Could you check a few things on this model? Use its own coordinates, in mm. Give positions to 0.01 mm unless a question says otherwise; leave off trailing zeros. Loops run counter-clockwise (first coordinate to the right, second up) from the corner with the lowest first, then second, coordinate; pieces in that order, holes last. Notation, with made-up numbers: (76.5, 29.25) - (116.5, 29.25) arc R17 ccw to (116.5, 42.25) - close; hole circle Ø5 at (14, -2). An arc over 180 degrees is marked (long way). Write each question's results on one line, items separated by ' | '. Start each with the question number.
1) I want a section at A-A, the plane y = 92.5. Write out the boundary of the cut face in (x, z).
2) I'm going to push a flat-ended pin straight in: pin 1 (3 mm diameter, centred on y = 106.77, z = 239.43, fed in from +X). Where does the tip first touch, or does it pass through?
3) If we mould it in two halves opening along X, with no side actions, what happens to faces 1 (the face through (2, 75, 404.535)), 2 (the face through (4.762, 46, 295)), 3 (the face through (0, 46, 295))? For each: +X half, -X half, draft (parallel to the pull), parting line (faces both ways), or undercut.
4) I want a section at C-C, the plane x = 1.25. Count the separate pieces of the cut face and the enclosed holes in it, and give its area (3 significant figures).
5) I want a section at D-D, the plane y = 82.5. Write out the boundary of the cut face in (x, z), and give its area (3 significant figures).
6) If I drill on probe 1 along Z at (x, y) = (3.6, 42); probe 2 along Z at (x, y) = (2.7, 79); probe 3 along Z at (x, y) = (3.35, 88), over which ranges is the centre line in solid material (lowest first)? Write a range as [from, to].
7) I want a section at B-B, the plane z = 308. Write out the boundary of the cut face in (x, y), and give its area (3 significant figures).
from build123d import *

# Parameters (mm, degrees)
SKETCH1_R           = 2.54
SKETCH1_R_2         = 31.75
SKETCH1_R_3         = 9.525
BOSS_EXTRUDE1_DEPTH = 4.7625


with BuildPart() as part:
    # Sketch1 → Boss-Extrude1 (new body)
    with BuildSketch(Plane(origin=(0, 0, 0), x_dir=(0, 0, -1), z_dir=(1, 0, 0))):
        with BuildLine():
            Line((226.734866781, 43.274288567), (226.734866781, 106.774288567))
            ThreePointArc((226.734866781, 106.774288567), (230.45461066, 115.754544688), (239.434866781, 119.474288567))
            Line((239.434866781, 119.474288567), (391.834866781, 119.474288567))
            ThreePointArc((391.834866781, 119.474288567), (400.815122902, 115.754544688), (404.534866781, 106.774288567))
            Line((404.534866781, 106.774288567), (404.534866781, 43.274288567))
            ThreePointArc((404.534866781, 43.274288567), (400.815122902, 34.294032445), (391.834866781, 30.574288567))
            Line((391.834866781, 30.574288567), (239.434866781, 30.574288567))
            ThreePointArc((239.434866781, 30.574288567), (230.45461066, 34.294032445), (226.734866781, 43.274288567))
        make_face()
        with Locations(Location((302.934866781, 111.854288567, 0), (0, 0, 180))):
            Circle(SKETCH1_R, mode=Mode.SUBTRACT)
        with Locations(Location((328.334866781, 111.854288567, 0), (0, 0, 180))):
            Circle(SKETCH1_R, mode=Mode.SUBTRACT)
        with Locations(Location((302.934866781, 38.194288567, 0), (0, 0, 180))):
            Circle(SKETCH1_R, mode=Mode.SUBTRACT)
        with Locations(Location((328.334866781, 38.194288567, 0), (0, 0, 180))):
            Circle(SKETCH1_R, mode=Mode.SUBTRACT)
        with Locations(Location((239.434866781, 43.274288567, 0), (0, 0, 180))):
            Circle(SKETCH1_R, mode=Mode.SUBTRACT)
        with Locations(Location((391.834866781, 43.274288567, 0), (0, 0, 180))):
            Circle(SKETCH1_R, mode=Mode.SUBTRACT)
        with Locations(Location((315.634866781, 75.024288567, 0), (0, 0, 180))):
            Circle(SKETCH1_R_2, mode=Mode.SUBTRACT)
        with Locations(Location((239.434866781, 106.774288567, 0), (0, 0, 180))):
            Circle(SKETCH1_R, mode=Mode.SUBTRACT)
        with Locations(Location((391.834866781, 106.774288567, 0), (0, 0, 180))):
            Circle(SKETCH1_R, mode=Mode.SUBTRACT)
        with Locations(Location((269.914866781, 75.024288567, 0), (0, 0, 180))):
            Circle(SKETCH1_R_3, mode=Mode.SUBTRACT)
        with Locations(Location((361.354866781, 75.024288567, 0), (0, 0, 180))):
            Circle(SKETCH1_R_3, mode=Mode.SUBTRACT)
    extrude(amount=BOSS_EXTRUDE1_DEPTH)


with BuildPart() as part_1:
    # Body-Move/Copy1: moved
    add(part.part.moved(Location((0, 0, 631.269733563))))


solid = part_1.part
Answers:
1) outline: (0, 226.73) - (4.76, 226.73) - (4.76, 289.13) - (0, 289.13) - close; (0, 342.14) - (4.76, 342.14) - (4.76, 404.53) - (0, 404.53) - close
2) pin 1: passes through
3) face 1: draft | face 2: +X half | face 3: -X half
4) separate pieces: 1 | enclosed holes: 11 | area: 11,800 mm2
5) outline: (0, 226.73) - (4.76, 226.73) - (4.76, 264.01) - (0, 264.01) - close; (0, 275.82) - (4.76, 275.82) - (4.76, 284.78) - (0, 284.78) - close; (0, 346.49) - (4.76, 346.49) - (4.76, 355.45) - (0, 355.45) - close; (0, 367.26) - (4.76, 367.26) - (4.76, 404.53) - (0, 404.53) - close | area: 440 mm2
6) probe 1: z = [226.8, 237.24], [241.63, 389.64], [394.03, 404.47] | probe 2: z = [226.73, 261.26], [278.57, 284.13], [347.13, 352.7], [370.01, 404.53] | probe 3: z = [226.73, 286.66], [344.61, 404.53]
7) outline: (0, 30.57) - (4.76, 30.57) - (4.76, 44.21) - (0, 44.21) - close; (0, 105.84) - (4.76, 105.84) - (4.76, 119.47) - (0, 119.47) - close | area: 130 mm2
